Can you work these out from the model? Positions are in its coordinate system, mm. Round coordinates to 2 decimals unless told otherwise and drop trailing zeros. Loops run counter-clockwise (first coordinate to the right, second up) from the corner with the lowest first, then second, coordinate; pieces in that order, holes last. Notation, with made-up numbers: (-24, -6) -> (5, -6) arc R13 ccw to (5, 1) -> close; hole circle Ø6 at (72.25, 53.5). An arc over 180 degrees is marked (long way). Write item = value, one per line.
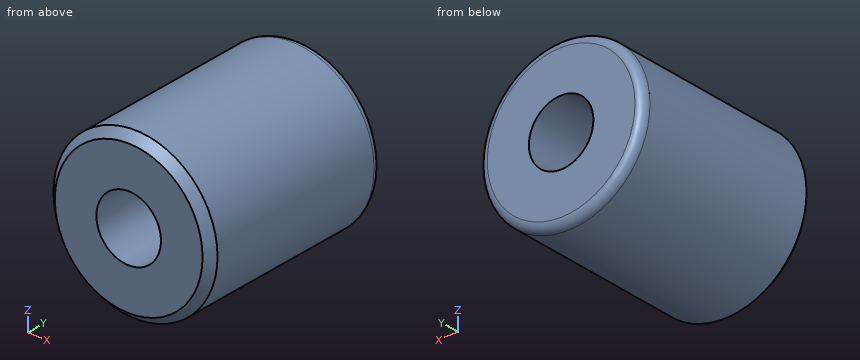
from build123d import *

# Parameters (mm, degrees)
F0_R     = 51.037505
F1_DEPTH = 63.5
F2_SIZE  = 5.08
F3_R     = 5.08
F4_R     = 20.080575
F5_DEPTH = 127.001


with BuildPart() as f1:
    # F0 (on Front) → F1 (new body, symmetric)
    with BuildSketch(Plane.XZ):
        Circle(F0_R)
    extrude(amount=F1_DEPTH, both=True)

    # F2
    f2_edges = [f1.edges().sort_by_distance(p)[0] for p in [
        (-51.037505, -63.5, 0),
    ]]
    chamfer(f2_edges, length=F2_SIZE)

    # F3
    f3_edges = [f1.edges().sort_by_distance(p)[0] for p in [
        (-51.037505, 63.5, 0),
    ]]
    fillet(f3_edges, radius=F3_R)

    # F4 (on face) → F5 (cut, through all)
    with BuildSketch(Plane(origin=(0, 63.5, 0), x_dir=(-1, 0, 0), z_dir=(0, 1, 0))):
        Circle(F4_R)
    extrude(amount=-F5_DEPTH, mode=Mode.SUBTRACT)


solid = f1.part
1. Suppose I cut it at B-B, the plane z = 0. List the corners of the cut face in (x, y) for me.
Entries:
outline = (-51.04, -58.42) -> (-45.96, -63.5) -> (-20.08, -63.5) -> (-20.08, 63.5) -> (-45.96, 63.5) arc R5.08 ccw to (-51.04, 58.42) -> close; (20.08, -63.5) -> (45.96, -63.5) -> (51.04, -58.42) -> (51.04, 58.42) arc R5.08 ccw to (45.96, 63.5) -> (20.08, 63.5) -> close
2. I need wall thicknesses on line 1 (Z direction, x = 0, y = 19.5); line 2 (Z direction, x = -3.5, y = 30); line 3 (X direction, y = 48.5, z = 14). Which ranges of each line are inside material? Lowest first, please. Write a range as [from, to].
Entries:
line_1 = [-51.04, -20.08], [20.08, 51.04]
line_2 = [-50.92, -19.77], [19.77, 50.92]
line_3 = [-49.08, -14.4], [14.4, 49.08]
3. Suppose I cut it at A-A, the plane x = 0. List the corners of the cut face in (y, z) for me.
Entries:
outline = (-63.5, -45.96) -> (-58.42, -51.04) -> (58.42, -51.04) arc R5.08 ccw to (63.5, -45.96) -> (63.5, -20.08) -> (-63.5, -20.08) -> close; (-63.5, 20.08) -> (63.5, 20.08) -> (63.5, 45.96) arc R5.08 ccw to (58.42, 51.04) -> (-58.42, 51.04) -> (-63.5, 45.96) -> close
4. I'm going to push flat-ended pins straight in: pin 1 (12 mm diameter, centred on x = -26, y = -24, fed in from -Z); pin 2 (4 mm diameter, centred on y = 5, z = -28.5, fed in from +X); pin 3 (10 mm diameter, centred on x = 3, y = 50, fed in from -Z). Where does each tip first touch, or does it pass through?
Entries:
pin_1 = -46.96
pin_2 = 43.62
pin_3 = -51.04
5. Suppose I cut it at C-C, the plane y = 53. List the corners of the cut face in (x, z) for me.
Entries:
outline = circle Ø102.08 at (0, 0); hole circle Ø40.16 at (0, 0)
